Work out the finished part from the listing and answer in its coordinate system (mm). A direction names the side the tool comes from. Round coordinates to 2 decimals unless told otherwise and drop trailing zeros. Write each loop counter-clockwise with the first axis right and the second up, starting at its lowest first coordinate (ties: lowest second). Pieces come first, ordered by that corner, then holes. Notation, with made-up numbers: (-4, -13) -> (13, -13) arc R16 cw to (13, 17) -> close; hole circle Ø3 at (-29.75, 88.5). An arc over 180 degrees is marked (long way). One line per item, written item: value.
Autodesk Inventor part; units mm, degrees
ref_plane "YZ Plane" through (0, 0, 0) normal (1, 0, 0) x (0, 1, 0)
ref_plane "XZ Plane" through (0, 0, 0) normal (0, 1, 0) x (-1, 0, 0)
ref_plane "XY Plane" through (0, 0, 0) normal (0, 0, 1) x (1, 0, 0)
sketch "Sketch1" plane through (0, 0, 0) normal (0, 1, 0) x (-1, 0, 0)
  line L0 (23.5034, -42.4981) -> (-1.8966, -42.4981)
  line L1 (-1.8966, -42.4981) -> (-1.8966, 770.3019)
  line L2 (-1.8966, 770.3019) -> (23.5034, 770.3019)
  line L3 (23.5034, 770.3019) -> (23.5034, -42.4981)
  line L4 (20.3284, -39.3231) -> (1.2784, -39.3231)
  line L5 (1.2784, -39.3231) -> (1.2784, 767.1269)
  line L6 (1.2784, 767.1269) -> (20.3284, 767.1269)
  line L7 (20.3284, 767.1269) -> (20.3284, -39.3231)
  point P0 (0, 0)
  dimension "d0" = 25.4
  dimension "d1" = 812.8
  dimension "d2" = 3.175
ref_plane "Work Plane3" through (0, 0, 0) normal (0, -1, 0) x (1, 0, 0)
sketch "Sketch2" plane through (0, 0, 0) normal (0, -1, 0) x (1, 0, 0)
  line L0 (-1.2784, -39.3231) -> (-20.3284, -39.3231)
  line L1 (-20.3284, -39.3231) -> (-20.3284, 767.1269)
  line L2 (-1.2784, -39.3231) -> (-20.3284, -39.3231)
  line L3 (-20.3284, -39.3231) -> (-20.3284, 767.1269)
  line L4 (-20.3284, 767.1269) -> (-1.2784, 767.1269)
  line L5 (-1.2784, 767.1269) -> (-1.2784, -39.3231)
  point P0 (0, 0)
extrude "Extrusion3" add sketch "Sketch2" against normal blind 3.175
extrude "Extrusion5" add sketch "Sketch1" along normal blind 50.8
sketch "Sketch4" plane through (-23.5034, 0, 770.3019) normal (0, 0, 1) x (1, 0, 0)
  line L0 (0, 50.8) -> (25.4, 50.8)
  line L1 (0, 50.8) -> (3.175, 50.8)
  line L2 (3.175, 50.8) -> (25.4, 50.8)
  line L3 (25.4, 50.8) -> (22.225, 50.8)
  line L4 (22.225, 3.175) -> (22.225, 50.8)
  line L5 (3.175, 50.8) -> (22.225, 50.8)
  line L6 (22.225, 50.8) -> (22.225, 3.175)
  line L7 (22.225, 3.175) -> (3.175, 3.175)
  line L8 (3.175, 3.175) -> (3.175, 50.8)
  point P0 (23.5034, 0)
  point P1 (22.225, 0)
  dimension "d13" = 3.175
  dimension "d14" = 3.175
extrude "Extrusion6" cut sketch "Sketch4" against normal blind 1016
sketch "Sketch5" plane through (1.8966, 0, 770.3019) normal (1, 0, 0) x (0, 0, -1)
  line L0 (0, 0) -> (19.05, 0)
  line L1 (19.05, 0) -> (19.05, 25.4)
  line L2 (19.05, 25.4) -> (0, 25.4)
  line L3 (0, 25.4) -> (0, 0)
  circle A0 centre (19.05, 25.4) radius 14.2875
  line L4 (19.05, 25.4) -> (76.2, 25.4)
  circle A1 centre (76.2, 25.4) radius 14.2875
  line L5 (76.2, 25.4) -> (107.95, 25.4)
  circle A2 centre (107.95, 25.4) radius 14.2875
  point P0 (770.3019, 0)
  dimension "d17" = 19.05
  dimension "d18" = 25.4
  dimension "d19" = 28.575
  dimension "d22" = 57.15
  dimension "d23" = 28.575
  dimension "d26" = 31.75
  dimension "d27" = 28.575
extrude "Extrusion10" cut sketch "Sketch5" against normal blind 50.8 contours A2 | A1 L5 L4 | L4 L5 A1 | A0 L2 L1 | L1 L4 A0 | A0 L4 L2
properties part number "36in Aluminum Channel"
(1) For a pull along Y with two mould halves and no side action, classify faces 3 (the face through (-21, 20, -42.498)), 4 (the face through (-21.894, 26.028, 765.526)), 5 (the face through (-11, 3.175, 370)) as pulls with the +Y half, pulls with the -Y half, needs draft (parallel to the pull), parting line crosses it, or undercut.
Reported:
face 3: needs draft
face 4: undercut
face 5: pulls with the +Y half
(2) Flat-ended cylindrical pins translate along their axes: pin 1 Ø17 at (y, z) = (25.4, 694.1) entering from +X; pin 2 Ø5 at (x, z) = (-11.5, 235) entering from -Y. Find the tip coordinate at first contact, or state that the pin passes through.
Reported:
pin 1: passes through
pin 2: stops at y = 0
(3) Consider probe 1 along Z at (x, y) = (-0.2, 25.4); probe 2 along X at (y, z) = (35.5, 192); probe 3 along Z at (x, y) = (0.25, 35.5). Determine where each line is inside the solid, lowest interval first.
Reported:
probe 1: z = -42.5 to 648.06, 676.64 to 679.81, 708.39 to 736.96, 765.54 to 770.3
probe 2: x = -23.5 to -20.33, -1.28 to 1.9
probe 3: z = -42.5 to 652.25, 672.46 to 684, 704.21 to 741.15, 761.36 to 770.3
(4) Find section C-C on x = -11.5. Give the vertices of the cut face in (y, z) (3 decimals), plus the area to 3 significant figures.
Reported:
outline: (0, -42.498) -> (3.175, -42.498) -> (3.175, 770.302) -> (0, 770.302) -> close
area: 2,580 mm2
(5) Find section B-B on z = 389.5. Give the vertices of the cut face in (x, y) (3 decimals).
Reported:
outline: (-23.503, 0) -> (1.897, 0) -> (1.897, 50.8) -> (-1.278, 50.8) -> (-1.278, 3.175) -> (-20.328, 3.175) -> (-20.328, 50.8) -> (-23.503, 50.8) -> close
(6) Find section A-A on y = 25.4. Give the number of separate pieces and of enclosed holes in the cut face, plus the area to 3 significant figures.
Reported:
separate pieces: 8
enclosed holes: 0
area: 4,620 mm2
(7) A tool of negligible diameter and unlimited length cuts with its end or side. For faces 1 (the face through (-11, 0, 370)), 2 (the face through (-20.328, 27, 370)), from which of +Z, -Z, +X, -X, +Y, -Y can it reach the whole face along a straight path? Write none if from no direction.
Reported:
face 1: +Z, -Z, +X, -X, -Y
face 2: +Z, -Z, +Y
